Source: CAD feature listing. Evaluate the final solid. Frame: model axes, mm. A direction names the side the tool comes from. Coordinates: 2 decimals unless noted, no trailing zeros. Write each loop counter-clockwise with the first axis right and the second up, starting at its lowest first coordinate (ties: lowest second). Pieces come first, ordered by that corner, then holes. Notation, with made-up numbers: M 81,61 L 129,61 A24 ccw 129,89 Z; hole C 69,68 d5. An arc over 180 degrees is marked long. One line per item, written item: value. Start each with the question number.
Item 1: Set-up query: faces 1 (the cylindrical face through (11.56, 40.35, 1.48)), 2 (the flat face through (145, 25, 2)). Return all of +Z, -Z, +X, -X, +Y, -Y with unobstructed straight access to the full face (end or side cutting, diameter ignored); none if empty.
Item 2: Mould query, pull axis X, two halves, no side actions, for faces 3 (the flat face through (0, 35, 1)), 4 (the cylindrical face through (48.92, 21.18, 1.48)), 5 (the flat face through (152, 0, 1)). Classes: released by +X, released by -X, zero draft, split by the parting line, or undercut.
Item 3: Cut plane C-C, the plane y = 20. Output: boundary loops of the cut face in (x, z).
Item 4: Cut plane D-D, the plane z = 2.3. State how many separate pieces and enclosed holes the cut face has, then the cut area to 3 significant figures.
Item 5: Cut plane B-B, the plane x = 10. Output: boundary loops of the cut face in (y, z), then the cut area to 3 significant figures.
Item 6: Cut plane A-A, the plane y = 29. Output: boundary loops of the cut face in (x, z), then the cut area to 3 significant figures.
Item 7: Ray query, L1, parallel to Y at x = 150, z = 2.05; L2, parallel to X at y = 20, z = 0.85; L3, parallel to X at y = 7.5, z = 2.1. Return the intervals inside material, ascending. Write a range as from..to.
Item 8: Pin query (flat end, axial travel): P1, Ø1, axis at x = 144, z = 2.5, coming from the -Y side; P2, Ø1.9, axis at x = 110, y = 20, coming from the -Z side. Return the tip coordinate at first contact, or that it passes through.
Autodesk Inventor part; units mm, degrees
ref_plane "YZ Plane" through (0, 0, 0) normal (1, 0, 0) x (0, 1, 0)
ref_plane "XZ Plane" through (0, 0, 0) normal (0, 1, 0) x (-1, 0, 0)
ref_plane "XY Plane" through (0, 0, 0) normal (0, 0, 1) x (1, 0, 0)
sketch "スケッチ1" plane through (0, 0, 0) normal (0, 0, 1) x (1, 0, 0)
  line L0 (0, 0) -> (160, 0)
  line L1 (160, 0) -> (160, 70)
  line L2 (160, 70) -> (0, 70)
  line L3 (0, 70) -> (0, 0)
  line L4 (20, 0) -> (40, 0)
  line L5 (40, 0) -> (40, 50)
  line L6 (40, 50) -> (20, 50)
  line L7 (20, 50) -> (20, 0)
  line L8 (140, 0) -> (120, 0)
  line L9 (120, 0) -> (120, 50)
  line L10 (120, 50) -> (140, 50)
  line L11 (140, 50) -> (140, 0)
  dimension "d0" = 70
  dimension "d1" = 160
  dimension "d2" = 20
  dimension "d3" = 20
  dimension "d4" = 50
  dimension "d5" = 20
  dimension "d6" = 20
  dimension "d7" = 50
extrude "押し出し1" add sketch "スケッチ1" along normal blind 3 contours L3 L2 L1 L0 L11 L10 L9 L5 L6 L7
sketch "スケッチ2" plane through (0, 0, 3) normal (0, 0, 1) x (1, 0, 0)
  line L0 (0, 70) -> (0, 0)
  line L1 (0, 0) -> (20, 0)
  line L2 (140, 0) -> (160, 0)
  line L3 (160, 0) -> (160, 70)
  point P0 (10, 10)
  point P1 (150, 10)
  point P2 (10, 40)
  point P3 (150, 40)
  dimension "d10" = 10
  dimension "d11" = 10
  dimension "d12" = 10
  dimension "d13" = 10
  dimension "d14" = 30
  dimension "d15" = 10
  dimension "d16" = 10
  dimension "d17" = 30
hole "穴1" at (10, 10, 3) at (150, 10, 3) at (10, 40, 3) at (150, 40, 3) direction (0, 0, -1) diameter 3.2 end through all
sketch "スケッチ3" plane through (0, 0, 3) normal (0, 0, 1) x (1, 0, 0)
  line L0 (0, 70) -> (0, 0)
  line L1 (160, 70) -> (0, 70)
  point P0 (30, 60)
  point P1 (130, 60)
  dimension "d25" = 30
  dimension "d26" = 10
  dimension "d27" = 10
  dimension "d28" = 100
hole "穴2" at (30, 60, 3) at (130, 60, 3) direction (0, 0, -1) diameter 3.2 end through all
sketch "スケッチ4" plane through (0, 0, 3) normal (0, 0, 1) x (1, 0, 0)
  line L0 (40, 0) -> (120, 0)
  line L1 (40, 50) -> (40, 0)
  line L2 (120, 0) -> (120, 50)
  point P0 (0, 0)
  point P1 (50, 20)
  point P2 (40, 25)
  point P3 (110, 20)
  dimension "d38" = 20
  dimension "d39" = 10
  dimension "d40" = 20
  dimension "d41" = 10
hole "穴3" at (50, 20, 3) at (110, 20, 3) direction (0, 0, -1) diameter 3.2 end through all
sketch "スケッチ5" plane through (0, 0, 3) normal (0, 0, 1) x (1, 0, 0)
  line L0 (20, 0) -> (20, 50)
  line L1 (20, 0) -> (15, 0)
  line L2 (15, 0) -> (15, 50)
  line L3 (15, 50) -> (20, 50)
  line L4 (20, 50) -> (20, 0)
  point P0 (0, 0)
  dimension "d49" = 50
  dimension "d50" = 5
extrude "押し出し2" cut sketch "スケッチ5" against normal blind 3
sketch "スケッチ6" plane through (0, 0, 3) normal (0, 0, 1) x (1, 0, 0)
  line L0 (140, 50) -> (140, 0)
  line L1 (140, 0) -> (145, 0)
  line L2 (145, 0) -> (145, 50)
  line L3 (145, 50) -> (140, 50)
  line L4 (140, 50) -> (140, 0)
  point P0 (0, 0)
  dimension "d53" = 50
  dimension "d54" = 5
extrude "押し出し3" cut sketch "スケッチ6" against normal blind 3
properties part number "backPlate" material "アルミニウム 6061"
From the geometry:
1. face 1: +Z, -Z
1. face 2: +Z, -Z, -Y
2. face 3: released by -X
2. face 4: undercut
2. face 5: zero draft
3. outline: M 0,0 L 15,0 L 15,3 L 0,3 Z; M 40,0 L 48.4,0 L 48.4,3 L 40,3 Z; M 51.6,0 L 108.4,0 L 108.4,3 L 51.6,3 Z; M 111.6,0 L 120,0 L 120,3 L 111.6,3 Z; M 145,0 L 160,0 L 160,3 L 145,3 Z
4. separate pieces: 1
4. enclosed holes: 8
4. area: 8,640 mm²
5. outline: M 0,0 L 8.4,0 L 8.4,3 L 0,3 Z; M 11.6,0 L 38.4,0 L 38.4,3 L 11.6,3 Z; M 41.6,0 L 70,0 L 70,3 L 41.6,3 Z
5. area: 191 mm²
6. outline: M 0,0 L 15,0 L 15,3 L 0,3 Z; M 40,0 L 120,0 L 120,3 L 40,3 Z; M 145,0 L 160,0 L 160,3 L 145,3 Z
6. area: 330 mm²
7. L1: y = 0..8.4, 11.6..38.4, 41.6..70
7. L2: x = 0..15, 40..48.4, 51.6..108.4, 111.6..120, 145..160
7. L3: x = 0..15, 40..120, 145..160
8. P1: stops at y = 50
8. P2: passes through
